```python
from build123d import *

# Parameters (mm, degrees)
F0_R          = 15
F2_ANGLE_BACK = 125
F2_ANGLE      = 250
F6_W          = 30
F6_H          = 50
F7_DEPTH      = 25
F9_W          = 20
F9_H          = 50
F7_FACE_W     = 30
F7_FACE_H     = 50


with BuildPart() as f2:
    # F0 (on Front) → F2 (revolve)
    with BuildSketch(Plane.XZ, mode=Mode.PRIVATE) as f2_sk:
        with Locations((105.5854605263, 0)):
            Circle(F0_R)
    revolve(f2_sk.sketch.rotate(Axis((-53.4410737455, 0, -2.1003899164), (0, 0, -1)), -F2_ANGLE_BACK), axis=Axis((-53.4410737455, 0, -2.1003899164), (0, 0, -1)), revolution_arc=F2_ANGLE)

    # F6 (on line) → F7 (join)
    with BuildSketch(Plane(origin=(1.8972807651, 0, -7.0807482116), x_dir=(0.9659258263, 0, 0.2588190451), z_dir=(0.2588190451, 0, -0.9659258263))):
        with Locations((87.3579102681, 0)):
            Rectangle(F6_W, F6_H)
    extrude(amount=F7_DEPTH)

    # F9 (on offset) → F10 section 0
    with BuildSketch(Plane(origin=(-49.8665282554, 0, 186.1044170462), x_dir=(0.9659258263, 0, 0.2588190451), z_dir=(0.2588190451, 0, -0.9659258263))):
        with Locations((86.933324366, -0.3083702177)):
            Rectangle(F9_W, F9_H)
    # F7_face (on face) → F10 section 1
    with BuildSketch(Plane(origin=(86.2785424237, 0, 15.5291427062), x_dir=(0.9659258263, 0, 0.2588190451), z_dir=(-0.2588190451, 0, 0.9659258263))):
        Rectangle(F7_FACE_W, F7_FACE_H)
    loft()


solid = f2.part
```
Work out the finished part from the listing and answer in its coordinate system (mm). A direction names the side the tool comes from. Round coordinates to 2 decimals unless told otherwise and drop trailing zeros. Loops run counter-clockwise (first coordinate to the right, second up) from the corner with the lowest first, then second, coordinate; pieces in that order, holes last.
(1) The mould has two halves that part along X. Classify faces 4 (the flat face through (85.637, -0.35, -10.525)), 5 (the flat face through (-144.53, 130.09, 0.21)), 6 (the flat face through (85, 25, 5)): pulls with the +X half, pulls with the -X half, needs draft (parallel to the pull), parting line crosses it, or undercut.
Computed values:
face 4: undercut
face 5: pulls with the -X half
face 6: needs draft
(2) The part is cut by section A-A, the plane x = 48.5. Give the number of separate pieces and of enclosed holes in the cut face, and give its area (3 significant figures).
Computed values:
separate pieces: 3
enclosed holes: 0
area: 6,250 mm2
(3) For faces 1 (the flat face through (74.98, 0.35, -0.26)), 2 (the flat face through (-144.53, -130.09, 0.21)), 3 (the flat face through (33.736, 0.562, 208.506)), determine the directions among +Z, -Z, +X, -X, +Y, -Y from which every point of the face is accessible in a straight line to the end or side of a thin tool.
Computed values:
face 1: -Z, -X
face 2: +Z, -Z, -X
face 3: +Z, -X, +Y, -Y
(4) Find the intervals of material crossed by L1, parallel to Y at x = -61.5, z = -2; L2, parallel to Z at x = 94, y = -58; L3, parallel to X at y = 23.5, z = 57, in increasing order.
Computed values:
L1: y = -173.71 to -143.94, 143.94 to 173.71
L2: z = -14.99 to 14.99
L3: x = 60.74 to 89.59
(5) The part is cut by section B-B, the plane z = 5.5. Give the vertices of the cut face in (x, y).
Computed values:
outline: (-152.66, -141.7) arc R172.98 ccw (long way) to (-152.66, 141.7) - (-136.65, 118.84) arc R145.07 cw to (89.46, 25) - (73.44, 25) - (73.44, -25) - (89.46, -25) arc R145.07 cw to (-136.65, -118.84) - close
(6) Each of these flat-tipped pins is pushed along its axis until it touches: P1, Ø9, axis at x = 91, z = -4, coming from the -Y side; P2, Ø9, axis at x = 90.5, z = 7.5, coming from the +Y side. Where does it stop, or does it pass through?
Computed values:
P1: stops at y = -102.79
P2: stops at y = 101.72
